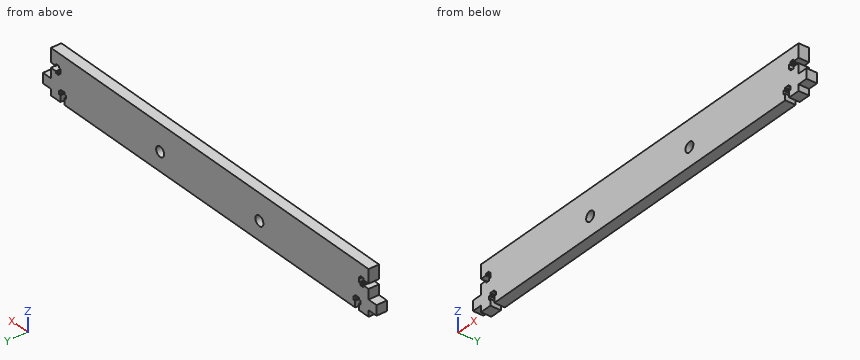
from build123d import *

# Parameters (mm, degrees)
SKETCH1_R           = 4
BOSS_EXTRUDE1_DEPTH = 8.4


with BuildPart() as part:
    # Sketch1 → Boss-Extrude1 (new body)
    with BuildSketch(Plane(origin=(0, 0, 0), x_dir=(1, 0, 0), z_dir=(0, 1, 0))):
        Polygon((-160, 18), (-150.5, 18), (-150.5, 13), (-152, 13), (-152, 10), (-150.5, 10), (-150.5, 8.5), (-146.5, 8.5), (-146.5, 10), (-145, 10), (-145, 13), (-146.5, 13), (-146.5, 18), (146.5, 18), (146.5, 13), (145, 13), (145, 10), (146.5, 10), (146.5, 8.5), (150.5, 8.5), (150.5, 10), (152, 10), (152, 13), (150.5, 13), (150.5, 18), (160, 18), (160, 13), (168, 13), (168, 5), (160, 5), (160, -3), (155, -3), (155, -1.5), (152, -1.5), (152, -3), (150.5, -3), (150.5, -7), (152, -7), (152, -8.5), (155, -8.5), (155, -7), (160, -7), (160, -18), (-160, -18), (-160, -7), (-155, -7), (-155, -8.5), (-152, -8.5), (-152, -7), (-150.5, -7), (-150.5, -3), (-152, -3), (-152, -1.5), (-155, -1.5), (-155, -3), (-160, -3), (-160, 5), (-168, 5), (-168, 13), (-160, 13), align=None)
        with Locations((-50, 3)):
            Circle(SKETCH1_R, mode=Mode.SUBTRACT)
        with Locations((50, 3)):
            Circle(SKETCH1_R, mode=Mode.SUBTRACT)
    extrude(amount=BOSS_EXTRUDE1_DEPTH)


solid = part.part
Geometry check sheet. Reference: the model listing, model coordinates, mm. Give positions to 0.01 mm unless a question says otherwise; leave off trailing zeros. Loops run counter-clockwise (first coordinate to the right, second up) from the corner with the lowest first, then second, coordinate; pieces in that order, holes last. Notation, with made-up numbers: (22.5, 30) -> (60.5, 30) arc R15 ccw to (60.5, 51) -> close; hole circle Ø9 at (-37.75, -18.5). An arc over 180 degrees is marked (long way). Answer in a Markdown table with one row per item. Add a question column.
1) Gauge pin test, flat ends, axial feed: P1, Ø1.6, axis at y = 5, z = 2, coming from the +X side; P2, Ø4, axis at y = 4, z = 7.5, coming from the -X side; P3, Ø4, axis at x = -165.5, y = 5, coming from the +Z side; P4, Ø12, axis at x = 43, z = 1.5, coming from the -Y side. Record the tip position at first contact, or that the pin passes through.
2) Cross-section at A-A on x = -50. Record the boundary of the cut face in (y, z).
3) Material ranges on probe 1 along X at (y, z) = (1.5, -3); probe 2 along X at (y, z) = (2.25, -9); probe 3 along Z at (x, y) = (-50, 4), recorded low to high. Write a range as from..to.
4) Cross-section at B-B on y = 5. State how many separate pieces and enclosed holes the cut face has, and give its area (3 significant figures).
Outcome:
| question | item | result |
|---|---|---|
| 1 | P1 | stops at x = 160 |
| 1 | P2 | stops at x = -160 |
| 1 | P3 | stops at z = -5 |
| 1 | P4 | stops at y = 0 |
| 2 | outline | (0, -18) -> (8.4, -18) -> (8.4, -7) -> (0, -7) -> close; (0, 1) -> (8.4, 1) -> (8.4, 18) -> (0, 18) -> close |
| 3 | probe 1 | x = -160..-54, -46..46, 54..160 |
| 3 | probe 2 | x = -168..-150.5, -146.5..146.5, 150.5..168 |
| 3 | probe 3 | z = -18..-7, 1..18 |
| 4 | separate pieces | 1 |
| 4 | enclosed holes | 2 |
| 4 | area | 11,400 mm^2 |
